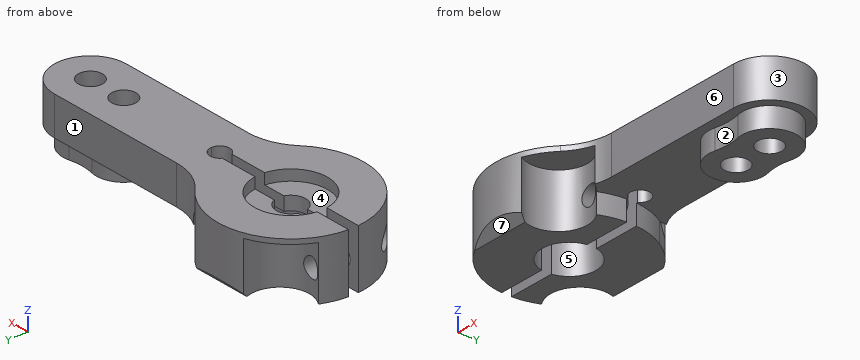
```python
from build123d import *

# Parameters (mm, degrees)
SKETCH_1_R               = 1.25
EXTRUDE_1_DEPTH          = 6
CUT_EXTRUDE_1_DEPTH      = 2.06
SKETCH_1_4_R             = 2.75
CUT_EXTRUDE_2_DEPTH      = 3.5
CUT_EXTRUDE_START        = 6
SKETCH_1_5_R             = 3.75
CUT_EXTRUDE_3_DEPTH      = 1.1
FILLET_1_R               = 6
SKETCH_2_R               = 3
CUT_EXTRUDE_4_DEPTH      = 5.5
CUT_EXTRUDE_5_DEPTH      = 30.317912613
CUT_EXTRUDE_5_DEPTH_BACK = 30.317912613
SKETCH_3_R               = 1
CUT_EXTRUDE_6_DEPTH      = 30.317912659
CUT_EXTRUDE_6_DEPTH_BACK = 30.317912659


with BuildPart() as part:
    # Эскиз1 → Бобышка-Вытянуть1 (new body)
    # profile 1 of 8: a face of its own
    with BuildSketch(Plane.XY):
        with BuildLine():
            ThreePointArc((24, -3.7), (27.7, 0), (24, 3.7))
            Line((24, 3.7), (6.523802572, 3.7))
            ThreePointArc((6.523802572, 3.7), (7.183998475, 2.154104435), (7.483314774, 0.5))
            Line((7.483314774, 0.5), (7.633974596, 0.5))
            ThreePointArc((7.633974596, 0.5), (8.758819045, 0.965925826), (9.5, 0))
            ThreePointArc((9.5, 0), (8.758819045, -0.965925826), (7.633974596, -0.5))
            Line((7.633974596, -0.5), (7.483314774, -0.5))
            ThreePointArc((7.483314774, -0.5), (7.183998475, -2.154104435), (6.523802572, -3.7))
            Line((6.523802572, -3.7), (24, -3.7))
        make_face()
        with BuildLine():
            ThreePointArc((23.363636364, 2.726727218), (26.8, 0), (23.363636364, -2.726727218))
            ThreePointArc((23.363636364, -2.726727218), (22, -2.569714114), (20.636363636, -2.726727218))
            ThreePointArc((20.636363636, -2.726727218), (17.2, 0), (20.636363636, 2.726727218))
            ThreePointArc((20.636363636, 2.726727218), (22, 2.569714114), (23.363636364, 2.726727218))
        make_face(mode=Mode.SUBTRACT)
    # profile 2 of 8: a face of its own
    with BuildSketch(Plane.XY):
        with BuildLine():
            ThreePointArc((20.636363636, 2.726727218), (22, 2.569714114), (23.363636364, 2.726727218))
            ThreePointArc((23.363636364, 2.726727218), (26.8, 0), (23.363636364, -2.726727218))
            ThreePointArc((23.363636364, -2.726727218), (22, -2.569714114), (20.636363636, -2.726727218))
            ThreePointArc((20.636363636, -2.726727218), (17.2, 0), (20.636363636, 2.726727218))
        make_face()
        with Locations((20, 0)):
            Circle(SKETCH_1_R, mode=Mode.SUBTRACT)
        with Locations((24, 0)):
            Circle(SKETCH_1_R, mode=Mode.SUBTRACT)
    # profile 3 of 8: a face of its own
    with BuildSketch(Plane.XY):
        with BuildLine():
            ThreePointArc((7.483314774, 0.5), (7.183998475, 2.154104435), (6.523802572, 3.7))
            ThreePointArc((6.523802572, 3.7), (-1.670378974, 7.311623218), (-7.483314774, 0.5))
            Line((-7.483314774, 0.5), (-3.716517187, 0.5))
            ThreePointArc((-3.716517187, 0.5), (0, 3.75), (3.716517187, 0.5))
            Line((3.716517187, 0.5), (7.483314774, 0.5))
        make_face()
    # profile 4 of 8: a face of its own
    with BuildSketch(Plane.XY):
        with BuildLine():
            ThreePointArc((3.716517187, 0.5), (0, 3.75), (-3.716517187, 0.5))
            Line((-3.716517187, 0.5), (-2.704163457, 0.5))
            ThreePointArc((-2.704163457, 0.5), (0, 2.75), (2.704163457, 0.5))
            Line((2.704163457, 0.5), (3.716517187, 0.5))
        make_face()
    # profile 5 of 8: a face of its own
    with BuildSketch(Plane.XY):
        with BuildLine():
            ThreePointArc((2.704163457, 0.5), (0, 2.75), (-2.704163457, 0.5))
            Line((-2.704163457, 0.5), (-1.414213562, 0.5))
            ThreePointArc((-1.414213562, 0.5), (0, 1.5), (1.414213562, 0.5))
            Line((1.414213562, 0.5), (2.704163457, 0.5))
        make_face()
    # profile 6 of 8: a face of its own
    with BuildSketch(Plane.XY):
        with BuildLine():
            ThreePointArc((-7.483314774, -0.5), (-1.670378974, -7.311623218), (6.523802572, -3.7))
            ThreePointArc((6.523802572, -3.7), (7.183998475, -2.154104435), (7.483314774, -0.5))
            Line((7.483314774, -0.5), (3.716517187, -0.5))
            ThreePointArc((3.716517187, -0.5), (0, -3.75), (-3.716517187, -0.5))
            Line((-3.716517187, -0.5), (-7.483314774, -0.5))
        make_face()
    # profile 7 of 8: a face of its own
    with BuildSketch(Plane.XY):
        with BuildLine():
            Line((-2.704163457, -0.5), (-3.716517187, -0.5))
            ThreePointArc((-3.716517187, -0.5), (0, -3.75), (3.716517187, -0.5))
            Line((3.716517187, -0.5), (2.704163457, -0.5))
            ThreePointArc((2.704163457, -0.5), (0, -2.75), (-2.704163457, -0.5))
        make_face()
    # profile 8 of 8: a face of its own
    with BuildSketch(Plane.XY):
        with BuildLine():
            Line((-1.414213562, -0.5), (-2.704163457, -0.5))
            ThreePointArc((-2.704163457, -0.5), (0, -2.75), (2.704163457, -0.5))
            Line((2.704163457, -0.5), (1.414213562, -0.5))
            ThreePointArc((1.414213562, -0.5), (0, -1.5), (-1.414213562, -0.5))
        make_face()
    extrude(amount=EXTRUDE_1_DEPTH)

    # Эскиз1<3> → Вырез-Вытянуть1 (cut)
    with BuildSketch(Plane.XY):
        with BuildLine():
            ThreePointArc((24, -3.7), (27.7, 0), (24, 3.7))
            Line((24, 3.7), (6.523802572, 3.7))
            ThreePointArc((6.523802572, 3.7), (7.183998475, 2.154104435), (7.483314774, 0.5))
            Line((7.483314774, 0.5), (7.633974596, 0.5))
            ThreePointArc((7.633974596, 0.5), (8.758819045, 0.965925826), (9.5, 0))
            ThreePointArc((9.5, 0), (8.758819045, -0.965925826), (7.633974596, -0.5))
            Line((7.633974596, -0.5), (7.483314774, -0.5))
            ThreePointArc((7.483314774, -0.5), (7.183998475, -2.154104435), (6.523802572, -3.7))
            Line((6.523802572, -3.7), (24, -3.7))
        make_face()
        with BuildLine():
            ThreePointArc((23.363636364, 2.726727218), (26.8, 0), (23.363636364, -2.726727218))
            ThreePointArc((23.363636364, -2.726727218), (22, -2.569714114), (20.636363636, -2.726727218))
            ThreePointArc((20.636363636, -2.726727218), (17.2, 0), (20.636363636, 2.726727218))
            ThreePointArc((20.636363636, 2.726727218), (22, 2.569714114), (23.363636364, 2.726727218))
        make_face(mode=Mode.SUBTRACT)
    extrude(amount=CUT_EXTRUDE_1_DEPTH, mode=Mode.SUBTRACT)

    # Эскиз1<4> → Вырез-Вытянуть2 (cut)
    with BuildSketch(Plane.XY):
        Circle(SKETCH_1_4_R)
    extrude(amount=CUT_EXTRUDE_2_DEPTH, mode=Mode.SUBTRACT)

    # Эскиз1<5> → Вырез-Вытянуть3 (cut)
    with BuildSketch(Plane.XY.offset(CUT_EXTRUDE_START)):
        Circle(SKETCH_1_5_R)
    extrude(amount=-CUT_EXTRUDE_3_DEPTH, mode=Mode.SUBTRACT)

    # Скругление1
    fillet_1_edges = [part.edges().sort_by_distance(p)[0] for p in [
        (6.523802572, 3.7, 4.03),
        (6.523802572, -3.7, 4.03),
    ]]
    fillet(fillet_1_edges, radius=FILLET_1_R)

    # Эскиз2 → Вырез-Вытянуть4 (cut)
    with BuildSketch(Plane.XY):
        with Locations((5.099019514, -5.5)):
            Circle(SKETCH_2_R)
        with Locations((-5.099019514, 5.5)):
            Circle(SKETCH_2_R)
    extrude(amount=CUT_EXTRUDE_4_DEPTH, mode=Mode.SUBTRACT)

    # Эскиз3 → Вырез-Вытянуть5 (cut, two sides: drawn at the far end of the back side and taken through both)
    with BuildSketch(Plane(origin=(0, 0, 0), x_dir=(1, 0, 0), z_dir=(0, 1, 0)).offset(-CUT_EXTRUDE_5_DEPTH_BACK)):
        with Locations(Location((5.5, -2.5, 0), (0, 0, 270))):
            Circle(SKETCH_3_R)
        with Locations(Location((-5.5, -2.5, 0), (0, 0, 270))):
            Circle(SKETCH_3_R)
    extrude(amount=CUT_EXTRUDE_5_DEPTH + CUT_EXTRUDE_5_DEPTH_BACK, mode=Mode.SUBTRACT)

    # Эскиз4 → Вырез-Вытянуть6 (cut, two sides: drawn at the far end of the back side and taken through both)
    with BuildSketch(Plane(origin=(0, 0, 0), x_dir=(0, 0, -1), z_dir=(1, 0, 0)).offset(-CUT_EXTRUDE_6_DEPTH_BACK)):
        Polygon((0, -6.5), (-1, -7.5), (0, -7.5), align=None)
        Polygon((0, 7.5), (0, 6.5), (-1, 7.5), align=None)
    extrude(amount=CUT_EXTRUDE_6_DEPTH + CUT_EXTRUDE_6_DEPTH_BACK, mode=Mode.SUBTRACT)


solid = part.part
```
Work out the finished part from the listing and answer in its coordinate system (mm). Face numbers are marked on the shaded views. A direction names the side the tool comes from. Coordinates: 2 decimals unless noted, no trailing zeros. Write each loop counter-clockwise with the first axis right and the second up, starting at its lowest first coordinate (ties: lowest second). Pieces come first, ordered by that corner, then holes.
Q1. Find the intervals of material crossed by line 1 (Y direction, x = 20, z = 1.55); line 2 (X direction, y = -1.8, z = 2.5); line 3 (Z direction, x = -5.5, y = 1.1), in increasing order.
Q2. A cutting plane is placed at B-B, the plane x = -5.5. Give the vertices of the cut face in (y, z).
Q3. A cutting plane is placed at D-D, the plane y = -4.75. Give the vertices of the cut face in (x, z), then the cut area to 3 significant figures.
Q4. Which of the six approach directions +Z, -Z, +X, -X, +Y, -Y give full straight-line access (tool end or side, diameter ignored) to the marked faces 5, 6 and 7?
Q5. A cutting plane is placed at A-A, the plane x = 20. Give the vertices of the cut face in (y, z), then the cut area to 3 significant figures.
Q6. Determine the mould class of the marked faces 1, 2, 3 and 4 for opening direction Y: released by +Y, released by -Y, zero draft, split by the parting line, or undercut.
Q7. Each of these flat-tipped pins is pushed along its axis until it touches: pin 1 Ø3 at (x, z) = (20, 3.5) entering from -Y; pin 2 Ø5 at (x, y) = (20, -4) entering from -Z; pin 3 Ø1.1 at (x, y) = (0.5, 1.5) entering from -Z; pin 4 Ø1 at (y, z) = (3, 5) entering from -X. Where does it stop, or does it pass through?
Q8. A cutting plane is placed at C-C, the plane z = 2.5. State how many separate pieces and enclosed holes the cut face has, then the cut area to 3 significant figures.
Findings below:
1. line 1: y = -2.8 to -1.25, 1.25 to 2.8
1. line 2: x = -7.28 to -6.5, -4.5 to -2.08, 2.08 to 4.5, 6.5 to 27.23
1. line 3: z = 0 to 1.5, 3.5 to 6
2. outline: (-5.1, 0) - (-0.5, 0) - (-0.5, 1.5) - (-5.1, 1.5) - close; (-5.1, 3.5) - (-0.5, 3.5) - (-0.5, 6) - (-5.1, 6) - close; (0.5, 0) - (2.53, 0) - (2.53, 1.5) - (0.5, 1.5) - close; (0.5, 3.5) - (2.53, 3.5) - (2.53, 5.5) - (5.1, 5.5) - (5.1, 6) - (0.5, 6) - close
3. outline: (-5.8, 0) - (2.19, 0) - (2.19, 5.5) - (6, 5.5) - (6, 6) - (-5.8, 6) - (-5.8, 3.45) arc R1 cw (long way) to (-5.8, 1.55) - close
3. area: 47.7 mm2
4. face 5: -Z
4. face 6: +Z, -Z, +X, -Y
4. face 7: -Z, +X, -X, -Y
5. outline: (-3.7, 2.06) - (-2.8, 2.06) - (-2.8, 0) - (-1.25, 0) - (-1.25, 6) - (-3.7, 6) - close; (1.25, 0) - (2.8, 0) - (2.8, 2.06) - (3.7, 2.06) - (3.7, 6) - (1.25, 6) - close
5. area: 25.7 mm2
6. face 1: released by +Y
6. face 2: released by -Y
6. face 3: split by the parting line
6. face 4: undercut
7. pin 1: stops at y = -3.7
7. pin 2: stops at z = 0
7. pin 3: stops at z = 3.5
7. pin 4: stops at x = -7.07
8. separate pieces: 5
8. enclosed holes: 2
8. area: 225 mm2
